from build123d import *

# Parameters (mm, degrees)
CROQUIS2_W                      = 20
CROQUIS2_H                      = 17
SALIENTE_EXTRUIR1_DEPTH         = 1.5
CROQUIS3_W                      = 20
CROQUIS3_H                      = 17
SALIENTE_EXTRUIR2_DEPTH         = 3
RANURA_START                    = -1.5
RANURA_DE_MARGEN_PARA_M65_DEPTH = 3
REDONDEO1_R                     = 0.5
SALIENTE_EXTRUIR3_DEPTH         = 3
TALADRO_DE_MARGEN_PARA_M51_D    = 5.3
SALIENTE_EXTRUIR4_DEPTH         = 5
REDONDEO2_R                     = 0.5


# Read off the part's stored shape, not the designer's step: Ranura de margen para M65
with BuildPart() as part:
    # Croquis2 → Saliente-Extruir1 (new, symmetric)
    with BuildSketch(Plane.XY):
        Rectangle(CROQUIS2_W, CROQUIS2_H)
    extrude(amount=SALIENTE_EXTRUIR1_DEPTH, both=True)

    # Croquis3 → Saliente-Extruir2 (add)
    with BuildSketch(Plane(origin=(7, 0, 0), x_dir=(0, 0, -1), z_dir=(1, 0, 0))):
        with Locations((-8.5, 0)):
            Rectangle(CROQUIS3_W, CROQUIS3_H)
    extrude(amount=SALIENTE_EXTRUIR2_DEPTH)

    # Ranura de margen para M65 outline → Ranura de margen para M65 (cut)
    with BuildSketch(Plane.XY.offset(RANURA_START)):
        with BuildLine():
            Line((-2.5, -3), (0.5, -3))
            ThreePointArc((0.5, -3), (3.5, 0), (0.5, 3))
            Line((0.5, 3), (-2.5, 3))
            ThreePointArc((-2.5, 3), (-5.5, 0), (-2.5, -3))
        make_face()
    extrude(amount=RANURA_DE_MARGEN_PARA_M65_DEPTH, mode=Mode.SUBTRACT)

    # Redondeo1
    redondeo1_edges = [part.edges().sort_by_distance(p)[0] for p in [
        (7, 0, 1.5),
    ]]
    fillet(redondeo1_edges, radius=REDONDEO1_R)

    # Croquis9 → Saliente-Extruir3 (add)
    with BuildSketch(Plane.XZ.offset(8.5)):
        Polygon((7, 18.5), (-10, 1.5), (-10, -1.5), (10, -1.5), (10, 18.5), align=None)
    saliente_extruir3 = extrude(amount=-SALIENTE_EXTRUIR3_DEPTH)

    # Simetría2: Saliente-Extruir3 across plane
    add(saliente_extruir3.mirror(Plane.ZX))

    # Taladro de margen para M51 (through all)
    with Locations(Plane.ZY.offset(-7)):
        with Locations((9.5, 0)):
            Hole(TALADRO_DE_MARGEN_PARA_M51_D / 2)

    # Croquis12 → Saliente-Extruir4 (add)
    with BuildSketch(Plane(origin=(10, 0, 0), x_dir=(0, 0, -1), z_dir=(1, 0, 0))):
        Polygon((-6.007030871, -6.05), (-2.514061743, 0), (-6.007030871, 6.05), (-12.992969129, 6.05), (-16.485938257, 0), (-12.992969129, -6.05), align=None)
        Polygon((-7.16173141, -4.05), (-4.82346282, 0), (-7.16173141, 4.05), (-11.83826859, 4.05), (-14.17653718, 0), (-11.83826859, -4.05), align=None, mode=Mode.SUBTRACT)
    extrude(amount=SALIENTE_EXTRUIR4_DEPTH)

    # Redondeo2
    redondeo2_edges = [part.edges().sort_by_distance(p)[0] for p in [
        (15, -6.05, 9.5),
        (15, -3.025, 4.260546307),
        (15, 3.025, 4.260546307),
        (15, 6.05, 9.5),
        (15, 3.025, 14.739453693),
        (15, -3.025, 14.739453693),
        (10, -6.05, 9.5),
        (12.5, -6.05, 12.992969129),
        (10, -3.025, 4.260546307),
        (12.5, -6.05, 6.007030871),
        (10, 3.025, 4.260546307),
        (12.5, 0, 2.514061743),
        (10, 6.05, 9.5),
        (12.5, 6.05, 6.007030871),
        (10, 3.025, 14.739453693),
        (12.5, 6.05, 12.992969129),
        (10, -3.025, 14.739453693),
        (12.5, 0, 16.485938257),
    ]]
    fillet(redondeo2_edges, radius=REDONDEO2_R)


solid = part.part
Build history of the part. All positions in model axes, mm. A direction names the side the tool comes from. Give positions to 0.01 mm unless a question says otherwise; leave off trailing zeros. Order: outer loops, then holes, each group sorted by start corner. A loop starts at its lowest first (then second) coordinate and runs counter-clockwise, first axis right, second up. Notation, with made-up numbers: M 5.25,21 L 45.25,21 A23 ccw 45.25,29 Z; hole C 13,-9 d7. An arc over 180 degrees is marked long. Put each result on its own line as item: value.
Item 1: Cut at A-A on z = 9.5. Write the cut outline in (x, y).
Results are:
outline: M -2,-8.5 L 10,-8.5 L 10,-6.55 A0.5 cw 10.5,-6.05 L 14.5,-6.05 A0.5 ccw 15,-5.55 L 15,-4.05 L 10,-4.05 L 10,-2.65 L 7,-2.65 L 7,-5.5 L -2,-5.5 Z; M -2,5.5 L 7,5.5 L 7,2.65 L 10,2.65 L 10,4.05 L 15,4.05 L 15,5.55 A0.5 ccw 14.5,6.05 L 10.5,6.05 A0.5 cw 10,6.55 L 10,8.5 L -2,8.5 Z
Item 2: Cut at D-D on x = 11.75. Write the cut outline in (y, z).
Results are:
outline: M -6.05,6.3 A0.5 ccw -5.8,5.86 L -0.25,2.66 A0.5 ccw 0.25,2.66 L 5.8,5.86 A0.5 ccw 6.05,6.3 L 6.05,12.7 A0.5 ccw 5.8,13.14 L 0.25,16.34 A0.5 ccw -0.25,16.34 L -5.8,13.14 A0.5 ccw -6.05,12.7 Z; hole M -4.05,7.16 L 0,4.82 L 4.05,7.16 L 4.05,11.84 L 0,14.18 L -4.05,11.84 Z
Item 3: Cut at B-B on z = 0. Write the cut outline in (x, y).
Results are:
outline: M -10,-8.5 L 10,-8.5 L 10,8.5 L -10,8.5 Z; hole M -2.5,-3 L 0.5,-3 A3 ccw 0.5,3 L -2.5,3 A3 ccw Z
Item 4: Wall check: probe 1 along Y at (x, z) = (-1.75, 7.5); probe 2 along Y at (x, z) = (-1.25, -0.5); probe 3 along X at (y, z) = (-5, 10.5). Give the ranges that are in metal, low to high.
Results are:
probe 1: -8.5 to -5.5, 5.5 to 8.5
probe 2: -8.5 to -3, 3 to 8.5
probe 3: 7 to 15
Item 5: Drop flat-ended pins along their axis: pin 1 Ø4.5 at (x, z) = (12.5, 10.5) entering from -Y; pin 2 Ø1.5 at (y, z) = (0, 12) entering from +X; pin 3 Ø3.5 at (x, z) = (12, 10) entering from +Y. Give the stop position or say it passes through.
Results are:
pin 1: y = -6.12
pin 2: x = 10
pin 3: y = 6.12
Item 6: Cut at C-C on x = -7. Write the cut outline in (y, z), then the cut area to 3 significant figures.
Results are:
outline: M -8.5,-1.5 L 8.5,-1.5 L 8.5,4.5 L 5.5,4.5 L 5.5,1.5 L -5.5,1.5 L -5.5,4.5 L -8.5,4.5 Z
area: 69.0 mm2
Item 7: Which spindle directions (+Z, -Z, +X, -X, +Y, -Y) get a long thin tool onto all of the face, cutting with end or side? Do faces 4 (the face through (12.47, -2.99, 14.76)), 5 (the face through (12.47, 2.99, 4.24)), 6 (the face through (12.46, 2, 5.98)), 7 (the face through (12.47, -3.06, 4.28)). Say none if no direction does.
Results are:
face 4: +Z, +X, -Y
face 5: -Z, +X, +Y
face 6: +X
face 7: -Z, +X, -Y
Item 8: Pull direction Z, two halves, no side cores. Call faces 1 (the face through (2, -8.5, 6)), 2 (the face through (8.521, 0.117, 12.147)), 3 (the face through (14.85, 2.993, 4.406)): +Z half, -Z half, draft (parallel to the pull), parting line (faces both ways), or undercut.
Results are:
face 1: draft
face 2: undercut
face 3: -Z half
